Input: part model. Units: mm. Frame: model coordinates. A direction names the side the tool comes from. Round coordinates to 2 decimals unless told otherwise and drop trailing zeros. Loops run counter-clockwise (first coordinate to the right, second up) from the corner with the lowest first, then second, coordinate; pieces in that order, holes last. Notation, with made-up numbers: (-24.5, 85.5) -> (24.5, 85.5) arc R17 cw to (24.5, 113.5) -> close; hole circle Ø3 at (50.5, 1). An arc over 180 degrees is marked (long way). Answer as a JSON object with one key per item and string values.
```python
from build123d import *

# Parameters (mm, degrees)
F1_DEPTH = 203.2
F2_DEPTH = 101.6


with BuildPart() as f1:
    # F0 (on Top) → F1 (new body)
    with BuildSketch(Plane.XY):
        with BuildLine():
            ThreePointArc((37.909021, -3.81), (38.052225, -1.907392), (38.1, 0))
            ThreePointArc((38.1, 0), (38.052225, 1.907392), (37.909021, 3.81))
            Line((37.909021, 3.81), (31.115, 3.81))
            Line((31.115, 3.81), (31.115, -3.81))
            Line((31.115, -3.81), (37.909021, -3.81))
        make_face()
        with BuildLine():
            Line((-31.115, 3.81), (-37.909021, 3.81))
            ThreePointArc((-37.909021, 3.81), (-38.1, 0), (-37.909021, -3.81))
            Line((-37.909021, -3.81), (-31.115, -3.81))
            Line((-31.115, -3.81), (-31.115, 3.81))
        make_face()
        with BuildLine():
            Line((3.81, 31.115), (3.81, 37.909021))
            ThreePointArc((3.81, 37.909021), (0, 38.1), (-3.81, 37.909021))
            Line((-3.81, 37.909021), (-3.81, 31.115))
            Line((-3.81, 31.115), (3.81, 31.115))
        make_face()
        with BuildLine():
            ThreePointArc((-3.81, -37.909021), (0, -38.1), (3.81, -37.909021))
            Line((3.81, -37.909021), (3.81, -31.115))
            Line((3.81, -31.115), (-3.81, -31.115))
            Line((-3.81, -31.115), (-3.81, -37.909021))
        make_face()
        with BuildLine():
            Line((31.115, 3.81), (37.909021, 3.81))
            ThreePointArc((37.909021, 3.81), (26.940768, 26.940768), (3.81, 37.909021))
            Line((3.81, 37.909021), (3.81, 31.115))
            Line((3.81, 31.115), (-3.81, 31.115))
            Line((-3.81, 31.115), (-3.81, 37.909021))
            ThreePointArc((-3.81, 37.909021), (-26.940768, 26.940768), (-37.909021, 3.81))
            Line((-37.909021, 3.81), (-31.115, 3.81))
            Line((-31.115, 3.81), (-31.115, -3.81))
            Line((-31.115, -3.81), (-37.909021, -3.81))
            ThreePointArc((-37.909021, -3.81), (-26.940768, -26.940768), (-3.81, -37.909021))
            Line((-3.81, -37.909021), (-3.81, -31.115))
            Line((-3.81, -31.115), (3.81, -31.115))
            Line((3.81, -31.115), (3.81, -37.909021))
            ThreePointArc((3.81, -37.909021), (26.940768, -26.940768), (37.909021, -3.81))
            Line((37.909021, -3.81), (31.115, -3.81))
            Line((31.115, -3.81), (31.115, 3.81))
        make_face()
    extrude(amount=F1_DEPTH)

    # F0 (on Top) → F2 (join)
    with BuildSketch(Plane.XY):
        with BuildLine():
            ThreePointArc((-37.909021, -3.81), (-38.1, 0), (-37.909021, 3.81))
            Line((-37.909021, 3.81), (-45.085, 3.81))
            Line((-45.085, 3.81), (-45.085, -3.81))
            Line((-45.085, -3.81), (-37.909021, -3.81))
        make_face()
        with BuildLine():
            Line((3.81, -45.085), (3.81, -37.909021))
            ThreePointArc((3.81, -37.909021), (0, -38.1), (-3.81, -37.909021))
            Line((-3.81, -37.909021), (-3.81, -45.085))
            Line((-3.81, -45.085), (3.81, -45.085))
        make_face()
        with BuildLine():
            ThreePointArc((37.909021, 3.81), (38.052225, 1.907392), (38.1, 0))
            ThreePointArc((38.1, 0), (38.052225, -1.907392), (37.909021, -3.81))
            Line((37.909021, -3.81), (45.085, -3.81))
            Line((45.085, -3.81), (45.085, 3.81))
            Line((45.085, 3.81), (37.909021, 3.81))
        make_face()
        with BuildLine():
            ThreePointArc((-3.81, 37.909021), (0, 38.1), (3.81, 37.909021))
            Line((3.81, 37.909021), (3.81, 45.085))
            Line((3.81, 45.085), (-3.81, 45.085))
            Line((-3.81, 45.085), (-3.81, 37.909021))
        make_face()
    extrude(amount=F2_DEPTH)


solid = f1.part
```
1) Section A-A, the plane z = 172. Output: boundary loops of the cut face in (x, y).
Output:
{"outline": "(-37.91, -3.81) arc R38.1 ccw to (-3.81, -37.91) arc R38.1 ccw to (3.81, -37.91) arc R38.1 ccw to (37.91, -3.81) arc R38.1 ccw to (38.1, 0) arc R38.1 ccw to (37.91, 3.81) arc R38.1 ccw to (3.81, 37.91) arc R38.1 ccw to (-3.81, 37.91) arc R38.1 ccw to (-37.91, 3.81) arc R38.1 ccw to start"}
2) Section C-C, the plane y = -27.5. Output: boundary loops of the cut face in (x, z), plus the area to 3 significant figures.
Output:
{"outline": "(-26.37, 0) -> (26.37, 0) -> (26.37, 203.2) -> (-26.37, 203.2) -> close", "area": "10,700 mm^2"}
3) Reachability of faces 1 (the face through (-3.81, -41, 50)), 2 (the face through (-41, 3.81, 50)), 3 (the face through (-38.1, 0.1, 151.7)), 4 (the face through (3.81, 41, 50)), 5 (the face through (-0.1, -38.1, 151.7)) from +Z, -Z, +X, -X, +Y, -Y: full face, straight path, thin tool, end or side. Return the list, or none.
Output:
{"face 1": "+Z, -Z, -X, -Y", "face 2": "+Z, -Z, -X, +Y", "face 3": "+Z, -X", "face 4": "+Z, -Z, +X, +Y", "face 5": "+Z, -Y"}
4) Ray query, probe 1 along X at (y, z) = (-41, 9.5); probe 2 along Z at (x, y) = (-41, -3); probe 3 along Y at (x, z) = (-3.5, 169.5). Return the intervals inside material, ascending.
Output:
{"probe 1": "x = -3.81 to 3.81", "probe 2": "z = 0 to 101.6", "probe 3": "y = -37.94 to 37.94"}
5) Contact query for flat-ended pins moving along their axis: P1, Ø1, axis at x = -28, z = 52.5, coming from the -Y side; P2, Ø3.5, axis at y = -40.5, z = 48.5, coming from the +X side; P3, Ø5, axis at y = -26, z = 61.5, coming from the +X side. Output: stop coordinate, or through.
Output:
{"P1": "stops at y = -26.37", "P2": "stops at x = 3.81", "P3": "stops at x = 29.99"}
6) Section D-D, the plane z = 20. Output: boundary loops of the cut face in (x, y) (3 decimals).
Output:
{"outline": "(-45.085, -3.81) -> (-37.909, -3.81) arc R38.1 ccw to (-3.81, -37.909) -> (-3.81, -45.085) -> (3.81, -45.085) -> (3.81, -37.909) arc R38.1 ccw to (37.909, -3.81) -> (45.085, -3.81) -> (45.085, 3.81) -> (37.909, 3.81) arc R38.1 ccw to (3.81, 37.909) -> (3.81, 45.085) -> (-3.81, 45.085) -> (-3.81, 37.909) arc R38.1 ccw to (-37.909, 3.81) -> (-45.085, 3.81) -> close"}
7) Section B-B, the plane x = -1.5. Output: boundary loops of the cut face in (y, z) (3 decimals), plus the area to 3 significant figures.
Output:
{"outline": "(-45.085, 0) -> (45.085, 0) -> (45.085, 101.6) -> (38.07, 101.6) -> (38.07, 203.2) -> (-38.07, 203.2) -> (-38.07, 101.6) -> (-45.085, 101.6) -> close", "area": "16,900 mm^2"}
